Input: part model. Units: mm. Frame: model coordinates. Give positions to 0.01 mm unless a question says otherwise; leave off trailing zeros. Order: outer loops, then holes, each group sorted by start corner. A loop starts at its lowest first (then second) coordinate and runs counter-clockwise, first axis right, second up.
```python
from build123d import *

# Parameters (mm, degrees)
SKETCH1_R           = 127
BOSS_EXTRUDE1_DEPTH = 3.175
SKETCH2_W           = 127
SKETCH2_H           = 190.5
CUT_EXTRUDE1_DEPTH  = 3.175
SKETCH3_W           = 114.3
SKETCH3_H           = 32.385
BOSS_EXTRUDE2_DEPTH = 3.175
SKETCH4_W           = 101.6
SKETCH4_H           = 6.35
CUT_EXTRUDE2_DEPTH  = 3.175
SKETCH5_W           = 101.6
SKETCH5_H           = 3.175
BOSS_EXTRUDE5_DEPTH = 3.175
SKETCH6_W           = 114.3
SKETCH6_H           = 32.385
CUT_EXTRUDE3_DEPTH  = 4.175
SKETCH7_R           = 1.8288
CUT_EXTRUDE4_DEPTH  = 4.175
SKETCH8_W           = 6.35
SKETCH8_H           = 3.175
BOSS_EXTRUDE6_DEPTH = 3.175
SKETCH9_R           = 1.8288
CUT_EXTRUDE5_DEPTH  = 3.175
SKETCH10_R          = 1.8288
BOSS_EXTRUDE7_DEPTH = 3.175
CUT_EXTRUDE6_DEPTH  = 4.175
SKETCH13_W          = 3.175
SKETCH13_H          = 178.054
CUT_EXTRUDE8_DEPTH  = 4.175
SKETCH14_R          = 1.8288
CUT_EXTRUDE9_DEPTH  = 4.175
SKETCH15_W          = 133.858
SKETCH15_H          = 3.175
CUT_EXTRUDE10_DEPTH = 4.175
SKETCH16_R          = 1.8288
CUT_EXTRUDE11_DEPTH = 4.175
SKETCH17_R          = 1.8288
CUT_EXTRUDE12_DEPTH = 4.175


with BuildPart() as part:
    # Sketch1 → Boss-Extrude1 (new body)
    with BuildSketch(Plane(origin=(0, 0, 0), x_dir=(1, 0, 0), z_dir=(0, 1, 0))):
        Circle(SKETCH1_R)
    extrude(amount=BOSS_EXTRUDE1_DEPTH)

    # Sketch2 → Cut-Extrude1 (cut)
    with BuildSketch(Plane(origin=(0, 3.175, 0), x_dir=(1, 0, 0), z_dir=(0, 1, 0))):
        Rectangle(SKETCH2_W, SKETCH2_H)
    extrude(amount=-CUT_EXTRUDE1_DEPTH, mode=Mode.SUBTRACT)

    # Sketch3 → Boss-Extrude2 (add)
    with BuildSketch(Plane(origin=(0, 3.175, 0), x_dir=(1, 0, 0), z_dir=(0, 1, 0))):
        with Locations((0, -79.0575)):
            Rectangle(SKETCH3_W, SKETCH3_H)
    extrude(amount=-BOSS_EXTRUDE2_DEPTH)

    # Sketch4 → Cut-Extrude2 (cut)
    with BuildSketch(Plane.XZ):
        with Locations((0, 95.25)):
            Rectangle(SKETCH4_W, SKETCH4_H)
    extrude(amount=-CUT_EXTRUDE2_DEPTH, mode=Mode.SUBTRACT)

    # Sketch5 → Boss-Extrude5 (add, through all)
    with BuildSketch(Plane.XZ):
        with Locations((0, 93.6625)):
            Rectangle(SKETCH5_W, SKETCH5_H)
    extrude(amount=-BOSS_EXTRUDE5_DEPTH)

    # Sketch6 → Cut-Extrude3 (cut, through all)
    with BuildSketch(Plane.XZ):
        with Locations((0, 79.0575)):
            Rectangle(SKETCH6_W, SKETCH6_H)
    extrude(amount=-CUT_EXTRUDE3_DEPTH, mode=Mode.SUBTRACT)

    # Sketch7 → Cut-Extrude4 (cut, through all)
    with BuildSketch(Plane.XZ):
        with Locations((-47.752, 102.489)):
            Circle(SKETCH7_R)
        with Locations((-3.302, 102.489)):
            Circle(SKETCH7_R)
        with Locations((3.302, 102.489)):
            Circle(SKETCH7_R)
        with Locations((47.752, 102.489)):
            Circle(SKETCH7_R)
    extrude(amount=-CUT_EXTRUDE4_DEPTH, mode=Mode.SUBTRACT)

    # Sketch8 → Boss-Extrude6 (add)
    with BuildSketch(Plane.XZ):
        with Locations((-47.625, 96.8375)):
            Rectangle(SKETCH8_W, SKETCH8_H)
        with Locations((47.625, 96.8375)):
            Rectangle(SKETCH8_W, SKETCH8_H)
    extrude(amount=-BOSS_EXTRUDE6_DEPTH)

    # Sketch9 → Cut-Extrude5 (cut)
    with BuildSketch(Plane.XZ):
        with Locations((-41.402, 102.489)):
            Circle(SKETCH9_R)
        with Locations((41.402, 102.489)):
            Circle(SKETCH9_R)
    extrude(amount=-CUT_EXTRUDE5_DEPTH, mode=Mode.SUBTRACT)

    # Sketch10 → Boss-Extrude7 (add)
    with BuildSketch(Plane.XZ):
        with Locations((-47.752, 102.489)):
            Circle(SKETCH10_R)
        with Locations((47.752, 102.489)):
            Circle(SKETCH10_R)
    extrude(amount=-BOSS_EXTRUDE7_DEPTH)

    # Sketch11 → Cut-Extrude6 (cut, through all)
    with BuildSketch(Plane.XZ):
        Polygon((-63.754, 95.25), (-63.5, 95.25), (-63.5, -95.25), (63.5, -95.25), (63.5, 95.25), (63.754, 95.25), (63.754, -95.504), (-63.754, -95.504), align=None)
    extrude(amount=-CUT_EXTRUDE6_DEPTH, mode=Mode.SUBTRACT)

    # Sketch13 → Cut-Extrude8 (cut, through all)
    with BuildSketch(Plane.XZ):
        with Locations((-65.3415, -6.477)):
            Rectangle(SKETCH13_W, SKETCH13_H)
        with Locations((65.3415, -6.477)):
            Rectangle(SKETCH13_W, SKETCH13_H)
    extrude(amount=-CUT_EXTRUDE8_DEPTH, mode=Mode.SUBTRACT)

    # Sketch14 → Cut-Extrude9 (cut, through all)
    with BuildSketch(Plane.XZ):
        with Locations((-70.993, 79.502)):
            Circle(SKETCH14_R)
        with Locations((-70.993, -92.456)):
            Circle(SKETCH14_R)
        with Locations((-70.993, -3.429)):
            Circle(SKETCH14_R)
        with Locations((-70.993, -9.525)):
            Circle(SKETCH14_R)
        with Locations((70.993, -92.456)):
            Circle(SKETCH14_R)
        with Locations((70.993, -9.525)):
            Circle(SKETCH14_R)
        with Locations((70.993, -3.429)):
            Circle(SKETCH14_R)
        with Locations((70.993, 79.502)):
            Circle(SKETCH14_R)
    extrude(amount=-CUT_EXTRUDE9_DEPTH, mode=Mode.SUBTRACT)

    # Sketch15 → Cut-Extrude10 (cut, through all)
    with BuildSketch(Plane.XZ):
        with Locations((0, -97.0915)):
            Rectangle(SKETCH15_W, SKETCH15_H)
    extrude(amount=-CUT_EXTRUDE10_DEPTH, mode=Mode.SUBTRACT)

    # Sketch16 → Cut-Extrude11 (cut, through all)
    with BuildSketch(Plane.XZ):
        with Locations((-63.881, -102.743)):
            Circle(SKETCH16_R)
        with Locations((-3.048, -102.743)):
            Circle(SKETCH16_R)
        with Locations((3.048, -102.743)):
            Circle(SKETCH16_R)
        with Locations((63.881, -102.743)):
            Circle(SKETCH16_R)
    extrude(amount=-CUT_EXTRUDE11_DEPTH, mode=Mode.SUBTRACT)

    # Sketch17 → Cut-Extrude12 (cut, through all)
    with BuildSketch(Plane.XZ):
        with Locations((-70.993, 7.62)):
            Circle(SKETCH17_R)
        with Locations((-70.993, 58.42)):
            Circle(SKETCH17_R)
        with Locations((-70.993, 33.02)):
            Circle(SKETCH17_R)
        with Locations((70.993, 58.42)):
            Circle(SKETCH17_R)
        with Locations((70.993, 7.62)):
            Circle(SKETCH17_R)
        with Locations((70.993, 33.02)):
            Circle(SKETCH17_R)
    extrude(amount=-CUT_EXTRUDE12_DEPTH, mode=Mode.SUBTRACT)


solid = part.part
```
1) First-contact query: P1, Ø1.5, axis at y = 0.5, z = -35.5, coming from the -X side; P2, Ø1, axis at x = 23.5, y = 1.5, coming from the +Z side; P3, Ø1, axis at y = 2.5, z = 52.5, coming from the +X side. Flat tips, straight axial feed; report the tip coordinate or a pass-through.
2) Line query: probe 1 along X at (y, z) = (2.7, 1.5); probe 2 along X at (y, z) = (1.05, -8); probe 3 along Z at (x, y) = (-43, 2.55) (3 decimals). Output: solid intervals per line, ascending.
3) Cut plane C-C (x = -84). Return the cut outline in (y, z) (3 decimals), then the cut area to 3 significant figures.
4) Cut plane A-A (z = -50). Return the cut outline in (x, y) (3 decimals).
5) Cut plane B-B (x = 25.5). Return the cut outline in (y, z) (3 decimals), then the cut area to 3 significant figures.
6) Cut plane D-D (y = 2.15). Count the separate pieces of the cut face and the enclosed holes in it, then the cut area to 3 significant figures.
Geometry says:
1. P1: stops at x = -122.15
1. P2: stops at z = 124.9
1. P3: stops at x = 115.87
2. probe 1: x = -126.99 to -66.93, 66.93 to 126.99
2. probe 2: x = -126.75 to -72, -69.98 to -66.93, 66.93 to 69.98, 72 to 126.75
2. probe 3: z = -119.499 to -98.679, 98.425 to 101.6, 103.378 to 119.499
3. outline: (0, -95.252) - (3.175, -95.252) - (3.175, 95.252) - (0, 95.252) - close
3. area: 605 mm2
4. outline: (-116.743, 0) - (-66.929, 0) - (-66.929, 3.175) - (-116.743, 3.175) - close; (66.929, 0) - (116.743, 0) - (116.743, 3.175) - (66.929, 3.175) - close
5. outline: (0, -124.414) - (3.175, -124.414) - (3.175, -98.679) - (0, -98.679) - close; (0, 98.425) - (3.175, 98.425) - (3.175, 124.414) - (0, 124.414) - close
5. area: 164 mm2
6. separate pieces: 1
6. enclosed holes: 23
6. area: 24,300 mm2
